Source: CAD feature listing. Evaluate the final solid. Frame: model axes, mm. Face numbers are marked on the shaded views. A direction names the side the tool comes from. Round coordinates to 2 decimals unless told otherwise and drop trailing zeros. Return JSON: item names as keys, results as strings. Group by question number.
```python
from build123d import *

# Parameters (mm, degrees)
SKETCH_R             = 4
PAD_DEPTH            = 20
CYLINDER_R           = 26.62
CYLINDER_DEPTH       = 40
CYLINDER_ROLL_ANGLE  = 90.0000000001
CUT007_ROLL_ANGLE    = -20
CONE_PLACEMENT_ANGLE = 70
FILLET007_R          = 3


with BuildPart() as clone_of_pad:
    # Sketch → Pad (new body, symmetric)
    with BuildSketch(Plane.XZ):
        with Locations((0, 26.6209914966)):
            Circle(SKETCH_R)
        with Locations((14.3923946042, 22.395003144)):
            Circle(SKETCH_R)
        with Locations((24.2153056134, 11.0587595287)):
            Circle(SKETCH_R)
        with Locations((26.3500281875, -3.7885620995)):
            Circle(SKETCH_R)
        with Locations((20.1188029925, -17.4330420298)):
            Circle(SKETCH_R)
        with Locations((7.5, -25.5426542917)):
            Circle(SKETCH_R)
        with Locations((-7.5, -25.5426542917)):
            Circle(SKETCH_R)
        with Locations((-26.3500281875, -3.7885620995)):
            Circle(SKETCH_R)
        with Locations((-24.2153056134, 11.0587595287)):
            Circle(SKETCH_R)
        with Locations((-14.3923946042, 22.395003144)):
            Circle(SKETCH_R)
        with Locations((-20.1188029925, -17.4330420298)):
            Circle(SKETCH_R)
    extrude(amount=PAD_DEPTH, both=True)


with BuildPart() as cut007:
    # Cylinder → Cylinder (new body)
    with BuildSketch(Plane.XY):
        Circle(CYLINDER_R)
    extrude(amount=CYLINDER_DEPTH)


with BuildPart() as cut007_1:
    # Cylinder roll: moved
    add(cut007.part.rotate(Axis((0, 0, 0), (1, 0, 0)), CYLINDER_ROLL_ANGLE))


with BuildPart() as cut007_2:
    # Cylinder placement: moved
    add(cut007_1.part.moved(Location((0, 20, 0))))

    # Cut007: cut Clone of Pad
    add(clone_of_pad.part, mode=Mode.SUBTRACT)


with BuildPart() as cut007_3:
    # Cut007 roll: moved
    add(cut007_2.part.rotate(Axis((0, 0, 0), (1, 0, 0)), CUT007_ROLL_ANGLE))


with BuildPart() as cut007_4:
    # Cut007 placement: moved
    add(cut007_3.part)


with BuildPart() as fillet007:
    # Cone → Cone (revolve)
    with BuildSketch(Plane.XZ):
        Polygon((0, 0), (34, 0), (48.5, 40), (0, 40), align=None)
    revolve(axis=Axis((0, 0, 0), (0, 0, 1)))


with BuildPart() as fillet007_1:
    # Cone placement: moved
    add(fillet007.part.moved(Location((0, 18.7938524157, -6.8404028665))).rotate(Axis((0, 18.7938524157, -6.8404028665), (1, 0, 0)), CONE_PLACEMENT_ANGLE))

    # Cut008: cut Cut007
    add(cut007_4.part, mode=Mode.SUBTRACT)

    # Fillet007
    fillet007_edges = [fillet007_1.edges().sort_by_distance(p)[0] for p in [
        (-48.5, -18.793852, 6.840403),
        (-34, 18.793852, -6.840403),
    ]]
    fillet(fillet007_edges, radius=FILLET007_R)


with BuildPart() as part_mirroring005:
    # Part__Mirroring005: instance of Fillet007
    add(fillet007_1.part.mirror(Plane(origin=(0, 45, 0), x_dir=(1, 0, 0), z_dir=(0, 1, 0))))


solid = part_mirroring005.part
```
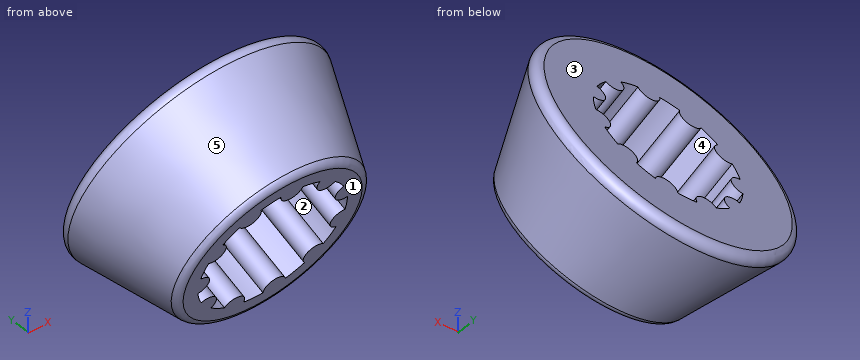
(1) Pin query (flat end, axial travel): pin 1 (5 mm diameter, centred on x = -17.5, y = 98.5, fed in from -Z); pin 2 (5 mm diameter, centred on y = 90, z = -28, fed in from +X); pin 3 (10 mm diameter, centred on x = -27.5, y = 68, fed in from +Z). Return the tip coordinate at first contact, or that it passes through.
(2) Ray query, line 1 (X direction, y = 111.5, z = -20); line 2 (X direction, y = 97, z = 9); line 3 (Z direction, x = -11, y = 82). Return the intervals inside material, ascending.
(3) Mould query, pull axis X, two halves, no side actions, for the marked faces 3, 4 and 5. Classes: released by +X, released by -X, zero draft, split by the parting line, or undercut.
(4) Set-up query: the marked faces 1 and 2. Return all of +Z, -Z, +X, -X, +Y, -Y with unobstructed straight access to the full face (end or side cutting, diameter ignored); none if empty.
Answers follow:
{
 "1": {"pin 1": "z = -36", "pin 2": "x = 29.64", "pin 3": "z = 24.69"},
 "2": {"line 1": "-37.96 to -3.55, 3.55 to 37.96", "line 2": "-44.34 to -25.92, 25.92 to 44.34", "line 3": "-35.95 to -28.03, 18.67 to 42.15"},
 "3": {"face 3": "zero draft", "face 4": "undercut", "face 5": "split by the parting line"},
 "4": {"face 1": "-Z, +X, -X, -Y", "face 2": "none"}
}
